```python
from build123d import *

# Parameters (mm, degrees)
SKETCH1_R           = 33
BOSS_EXTRUDE1_DEPTH = 3


with BuildPart() as part:
    # Sketch1 → Boss-Extrude1 (new body)
    with BuildSketch(Plane(origin=(0, 0, 0), x_dir=(1, 0, 0), z_dir=(0, 1, 0))):
        Circle(SKETCH1_R)
        with BuildLine():
            Line((-27, 3), (-22, 3))
            ThreePointArc((-22, 3), (-19.000055351, 0.018223725), (-21.963553222, -2.999778597))
            Line((-21.963553222, -2.999778597), (-27, -3))
            ThreePointArc((-27, -3), (-30, 0), (-27, 3))
        make_face(mode=Mode.SUBTRACT)
        with BuildLine():
            Line((-3, -27), (-3, -24))
            ThreePointArc((-3, -24), (0, -21), (3, -24))
            Line((3, -24), (3, -27))
            ThreePointArc((3, -27), (0, -30), (-3, -27))
        make_face(mode=Mode.SUBTRACT)
    extrude(amount=BOSS_EXTRUDE1_DEPTH)


solid = part.part
```
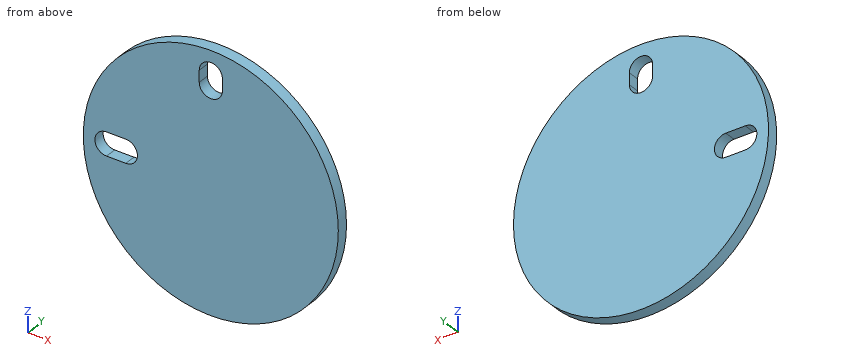
Can you work these out from the model? Positions are in its coordinate system, mm. Round coordinates to 2 decimals unless told otherwise and drop trailing zeros. Loops run counter-clockwise (first coordinate to the right, second up) from the corner with the lowest first, then second, coordinate; pieces in that order, holes last. Notation, with made-up numbers: M 77,5 L 119,5 A23 cw 119,41 Z; hole C 47.5,56.25 d2. An arc over 180 degrees is marked long. Write item = value, one per line. Start each with the question number.
(1) I need wall thicknesses on line 1 along X through (y, z) = (0.75, 1); line 2 along Z through (x, y) = (-29, 1.65); line 3 along Z through (x, y) = (-23.5, 2.9). Which ranges of each line are inside material? Lowest first, please.
(2) I'm going to push flat-ended pins straight in: P1, Ø1.5, axis at y = 2, z = -1.5, coming from the +X side; P2, Ø1.5, axis at x = 18, y = 0.5, coming from the -Z side; P3, Ø0.9, axis at y = 1, z = 25.5, coming from the +X side. Where does each tip first touch, or does it pass through?
(3) Suppose I cut it at C-C on y = 1.15. Write out the boundary of the cut face in (x, z).
(4) Suppose I cut it at D-D on z = 20. Write out the boundary of the cut face in (x, y), plus the area to 3 significant figures.
(5) Suppose I cut it at B-B on z = 0. Write out the boundary of the cut face in (x, y), plus the area to 3 significant figures.
(6) Suppose I cut it at A-A on x = 0. Write out the boundary of the cut face in (y, z), plus the area to 3 significant figures.
Answer block:
q1.line_1 = -32.98 to -29.83, -19.17 to 32.98
q1.line_2 = -15.75 to -2.24, 2.24 to 15.75
q1.line_3 = -23.17 to -3, 3 to 23.17
q2.P1 = 32.99
q2.P2 = -28.13
q2.P3 = 21.48
q3.outline = C 0,0 d66; hole M -27,-3 L -22,-3 A3 ccw -21.96,3 L -27,3 A3 ccw Z; hole M -3,24 A3 ccw 3,24 L 3,27 A3 ccw -3,27 Z
q4.outline = M -26.25,0 L 26.25,0 L 26.25,3 L -26.25,3 Z
q4.area = 157 mm²
q5.outline = M -33,0 L -30,0 L -30,3 L -33,3 Z; M -19,0 L 33,0 L 33,3 L -19,3 Z
q5.area = 165 mm²
q6.outline = M 0,-33 L 3,-33 L 3,21 L 0,21 Z; M 0,30 L 3,30 L 3,33 L 0,33 Z
q6.area = 171 mm²
